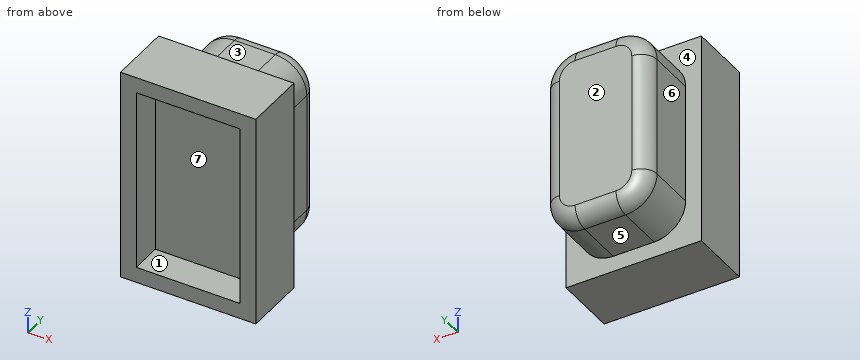
from build123d import *

# Parameters (mm, degrees)
EXTRUDE_1_DEPTH = 2
SKETCH_2_W      = 4.3
SKETCH_2_H      = 6.8
EXTRUDE_2_DEPTH = 1
SKETCH_4_W      = 4.3
SKETCH_4_H      = 6.8
SKETCH_4_W_2    = 3.3
SKETCH_4_H_2    = 5.8
EXTRUDE_3_DEPTH = 1
FILLET_1_R      = 0.5


with BuildPart() as part:
    # 草图1 → 凸台-拉伸1 (new body)
    with BuildSketch(Plane(origin=(0, 0, 0), x_dir=(1, 0, 0), z_dir=(0, 1, 0))):
        with BuildLine():
            Line((-0.65, -2.9), (0.65, -2.9))
            ThreePointArc((0.65, -2.9), (1.357106781, -2.607106781), (1.65, -1.9))
            Line((1.65, -1.9), (1.65, 1.9))
            ThreePointArc((1.65, 1.9), (1.357106781, 2.607106781), (0.65, 2.9))
            Line((0.65, 2.9), (-0.65, 2.9))
            ThreePointArc((-0.65, 2.9), (-1.357106781, 2.607106781), (-1.65, 1.9))
            Line((-1.65, 1.9), (-1.65, -1.9))
            ThreePointArc((-1.65, -1.9), (-1.357106781, -2.607106781), (-0.65, -2.9))
        make_face()
    extrude(amount=EXTRUDE_1_DEPTH)

    # 草图2 → 凸台-拉伸2 (add)
    with BuildSketch(Plane.XZ):
        Rectangle(SKETCH_2_W, SKETCH_2_H)
    extrude(amount=EXTRUDE_2_DEPTH)

    # 草图4 → 凸台-拉伸3 (add)
    with BuildSketch(Plane.XZ.offset(1)):
        Rectangle(SKETCH_4_W, SKETCH_4_H)
        Rectangle(SKETCH_4_W_2, SKETCH_4_H_2, mode=Mode.SUBTRACT)
    extrude(amount=EXTRUDE_3_DEPTH)

    # 圆角1
    fillet_1_edges = [part.edges().sort_by_distance(p)[0] for p in [
        (1.357106781, 2, -2.607106781),
        (0, 2, -2.9),
        (-1.357106781, 2, -2.607106781),
        (-1.65, 2, 0),
        (-1.357106781, 2, 2.607106781),
        (0, 2, 2.9),
        (1.357106781, 2, 2.607106781),
        (1.65, 2, 0),
    ]]
    fillet(fillet_1_edges, radius=FILLET_1_R)


solid = part.part
Part model, mm, in its own coordinate system. Face numbers are marked on the shaded views. A direction names the side the tool comes from. Round coordinates to 2 decimals unless told otherwise and drop trailing zeros. Write each loop counter-clockwise with the first axis right and the second up, starting at its lowest first coordinate (ties: lowest second). Pieces come first, ordered by that corner, then holes. Notation, with made-up numbers: M 86.5,26 L 138.5,26 A8 cw 138.5,37 Z; hole C 56.5,-27.5 d8. An arc over 180 degrees is marked long. Return JSON: item names as keys, results as strings. Group by question number.
(1) Two-plate mould, pull along Z, no slides. Class the marked faces 1, 2 and 3: +Z half, -Z half, draft (parallel to the pull), parting line (faces both ways), or undercut.
(2) Saw through at B-B on z = 0.25. Write the cut outline in (x, y), then the cut area to 3 significant figures.
(3) Saw through at C-C on x = 0.4. Write the cut outline in (y, z).
(4) Which spindle directions (+Z, -Z, +X, -X, +Y, -Y) get a long thin tool onto all of the face, cutting with end or side? Do the marked faces 4, 5, 6 and 7. Say none if no direction does.
(5) Drill centre lines: probe 1 along Z at (x, y) = (-0.8, -1.7); probe 2 along Y at (x, z) = (-0.55, 2); probe 3 along Y at (x, z) = (0.85, 3.25). Where is each one in solid material? Low to high.
(6) Saw through at D-D on y = 0.4. Write the cut outline in (x, z), then the cut area to 3 significant figures.
(7) Pin check, flat tips, straight feed: pin 1 Ø1.5 at (y, z) = (1, -2) entering from +X; pin 2 Ø0.8 at (y, z) = (1, 0.5) entering from -X; pin 3 Ø0.6 at (x, y) = (0, 0.5) entering from +Z. Stop position of each tip, or through.
(8) Saw through at A-A on y = -1.6. Write the cut outline in (x, z).
Returned:
{
 "1": {"face 1": "undercut", "face 2": "draft", "face 3": "+Z half"},
 "2": {"outline": "M -2.15,-2 L -1.65,-2 L -1.65,-1 L 1.65,-1 L 1.65,-2 L 2.15,-2 L 2.15,0 L 1.65,0 L 1.65,1.5 A0.5 ccw 1.15,2 L -1.15,2 A0.5 ccw -1.65,1.5 L -1.65,0 L -2.15,0 Z", "area": "11.8 mm²"},
 "3": {"outline": "M -2,-3.4 L 0,-3.4 L 0,-2.9 L 1.5,-2.9 A0.5 ccw 2,-2.4 L 2,2.4 A0.5 ccw 1.5,2.9 L 0,2.9 L 0,3.4 L -2,3.4 L -2,2.9 L -1,2.9 L -1,-2.9 L -2,-2.9 Z"},
 "4": {"face 4": "+Y", "face 5": "-Z, +X, -X, +Y", "face 6": "+Z, -Z, -X, +Y", "face 7": "-Y"},
 "5": {"probe 1": "-3.4 to -2.9, 2.9 to 3.4", "probe 2": "-1 to 2", "probe 3": "-2 to 0"},
 "6": {"outline": "M -1.65,-1.9 A1 ccw -0.65,-2.9 L 0.65,-2.9 A1 ccw 1.65,-1.9 L 1.65,1.9 A1 ccw 0.65,2.9 L -0.65,2.9 A1 ccw -1.65,1.9 Z", "area": "18.3 mm²"},
 "7": {"pin 1": "x = 1.65", "pin 2": "x = -1.65", "pin 3": "z = 2.9"},
 "8": {"outline": "M -2.15,-3.4 L 2.15,-3.4 L 2.15,3.4 L -2.15,3.4 Z; hole M -1.65,-2.9 L 1.65,-2.9 L 1.65,2.9 L -1.65,2.9 Z"}
}
